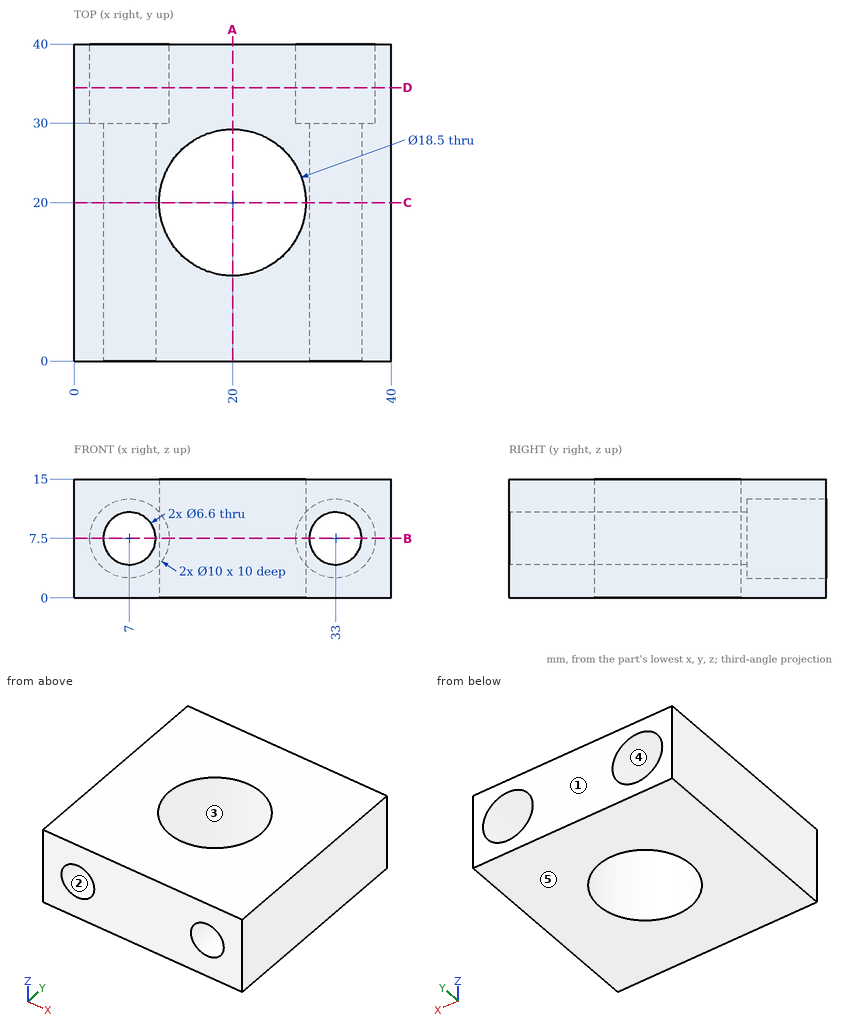
The drawing under review shows one solid part. Ordinate dimensions are in mm from its lowest x, y, z. A direction names the side the tool comes from. Round coordinates to 2 decimals unless told otherwise and drop trailing zeros. Write each loop counter-clockwise with the first axis right and the second up, starting at its lowest first coordinate (ties: lowest second). Pieces come first, ordered by that corner, then holes. Notation, with made-up numbers: (9.5, 75) -> (60.5, 75) arc R26 ccw to (60.5, 98) -> close; hole circle Ø2 at (67.25, 60). An arc over 180 degrees is marked (long way). Put each result on its own line as item: value.
Q1. Consider section B-B on z = 7.5. State the section outline as (x, y) points, and give its area (3 significant figures).
Determined:
outline: (0, 0) -> (3.7, 0) -> (3.7, 30) -> (2, 30) -> (2, 40) -> (0, 40) -> close; (10.3, 0) -> (29.7, 0) -> (29.7, 30) -> (28, 30) -> (28, 40) -> (12, 40) -> (12, 30) -> (10.3, 30) -> close; (36.3, 0) -> (40, 0) -> (40, 40) -> (38, 40) -> (38, 30) -> (36.3, 30) -> close; hole circle Ø18.5 at (20, 20)
area: 735 mm^2
Q2. To check wall thickness, follow L1, parallel to X at y = 31.5, z = 7.75; L2, parallel to Z at x = 7, y = 33.5; L3, parallel to Y at x = 20, z = 10.5. State the ranges of each line that lie inside material, in increasing order. Write a range as [from, to].
Determined:
L1: x = [0, 2.01], [11.99, 28.01], [37.99, 40]
L2: z = [0, 2.5], [12.5, 15]
L3: y = [0, 10.75], [29.25, 40]
Q3. Machinability: for the marked faces 4 and 5, which of the approach directions +Z, -Z, +X, -X, +Y, -Y give a long, thin tool a straight path to every point of the face, cutting with its end or side? Answer none if there is none.
Determined:
face 4: +Y
face 5: -Z, +X, -X, +Y, -Y
Q4. The part is to be moulded in two halves that separate along Y. For the marked faces 1, 2 and 3, say which applies: released by +Y, released by -Y, zero draft, split by the parting line, or undercut.
Determined:
face 1: released by +Y
face 2: zero draft
face 3: undercut
Q5. Consider section A-A on x = 20. State the section outline as (y, z) points.
Determined:
outline: (0, 0) -> (10.75, 0) -> (10.75, 15) -> (0, 15) -> close; (29.25, 0) -> (40, 0) -> (40, 15) -> (29.25, 15) -> close
Q6. Consider section D-D on y = 34.5. State the section outline as (x, z) points.
Determined:
outline: (0, 0) -> (40, 0) -> (40, 15) -> (0, 15) -> close; hole circle Ø10 at (7, 7.5); hole circle Ø10 at (33, 7.5)
Q7. Consider section C-C on y = 20. State the section outline as (x, z) points, and give its area (3 significant figures).
Determined:
outline: (0, 0) -> (10.75, 0) -> (10.75, 15) -> (0, 15) -> close; (29.25, 0) -> (40, 0) -> (40, 15) -> (29.25, 15) -> close; hole circle Ø6.6 at (7, 7.5); hole circle Ø6.6 at (33, 7.5)
area: 254 mm^2
Q8. Clearance check with a flat-ended pin moving along its axis: pin 1 Ø11 at (x, y) = (20, 20) entering from -Z. State where the tip first meets the part, or that it passes through.
Determined:
pin 1: passes through
